Can you work these out from the model? Positions are in its coordinate system, mm. A direction names the side the tool comes from. Give positions to 0.01 mm unless a question says otherwise; leave off trailing zeros. Order: outer loops, then holes, each group sorted by start corner. A loop starts at its lowest first (then second) coordinate and runs counter-clockwise, first axis right, second up. Notation, with made-up numbers: (72, -14) - (120, -14) arc R21 cw to (120, 9) - close; hole circle Ø3 at (-12.75, 1.5). An arc over 180 degrees is marked (long way). Answer as a JSON object with one key per item and string values.
```python
from build123d import *

# Parameters (mm, degrees)
F1_DEPTH = 1150
F2_W     = 1
F2_H     = 49
F3_DEPTH = 699
F4_W     = 1
F4_H     = 199
F5_DEPTH = 699


with BuildPart() as f1:
    # F0 (on Right) → F1 (new body)
    with BuildSketch(Plane.YZ):
        Polygon((699, 0), (0, 0), (0, -50), (1, -50), (1, -1), (700, -1), (700, 199), (699, 199), align=None)
    extrude(amount=-F1_DEPTH)

    # F2 (on face) → F3 (join, through all)
    with BuildSketch(Plane(origin=(0, 1, 0), x_dir=(-1, 0, 0), z_dir=(0, 1, 0))):
        with Locations((0.5, -25.5)):
            Rectangle(F2_W, F2_H)
    extrude(amount=F3_DEPTH)

    # F4 (on face) → F5 (join)
    with BuildSketch(Plane.XZ.offset(-699)):
        with Locations((-1149.5, 99.5)):
            Rectangle(F4_W, F4_H)
    extrude(amount=F5_DEPTH)


solid = f1.part
```
Q1. If we section it at B-B, the plane z = 129.5: Please give me the cut outline in (x, y).
Recorded:
{"outline": "(-1150, 0) - (-1149, 0) - (-1149, 699) - (0, 699) - (0, 700) - (-1150, 700) - close"}
Q2. If we section it at C-C, the plane y = 510: Please give me the cut outline in (x, z).
Recorded:
{"outline": "(-1150, -1) - (-1, -1) - (-1, -50) - (0, -50) - (0, 0) - (-1149, 0) - (-1149, 199) - (-1150, 199) - close"}
Q3. Which directions (+Z, -Z, +X, -X, +Y, -Y) give clear straight access to the entire face, cutting with the end or side of a thin tool? Please do faces 1 (the face through (-1, 346, -26)), 2 (the face through (-566, 354, 0)), 3 (the face through (-578, 0, -26)).
Recorded:
{"face 1": "-Z, -X, +Y", "face 2": "+Z, +X, -Y", "face 3": "+Z, -Z, +X, -X, -Y"}
Q4. If we section it at A-A, the plane x = -74.5: Please give me the cut outline in (y, z), then the cut area to 3 significant figures.
Recorded:
{"outline": "(0, -50) - (1, -50) - (1, -1) - (700, -1) - (700, 199) - (699, 199) - (699, 0) - (0, 0) - close", "area": "948 mm^2"}
Q5. I need wall thicknesses on L1, parallel to Y at x = -715, z = -19; L2, parallel to X at y = 399.5, z = 155.5; L3, parallel to Y at x = -1051, z = 10.5. Which ranges of each line are inside material? Lowest first, please.
Recorded:
{"L1": "y = 0 to 1", "L2": "x = -1150 to -1149", "L3": "y = 699 to 700"}
Q6. I'm going to push flat-ended pins straight in: pin 1 Ø8 at (x, z) = (-781.5, 118) entering from -Y; pin 2 Ø12 at (y, z) = (372.5, 78) entering from +X; pin 3 Ø1.5 at (x, y) = (-589, 128.5) entering from -Z. Where does each tip first touch, or does it pass through?
Recorded:
{"pin 1": "stops at y = 699", "pin 2": "stops at x = -1149", "pin 3": "stops at z = -1"}
